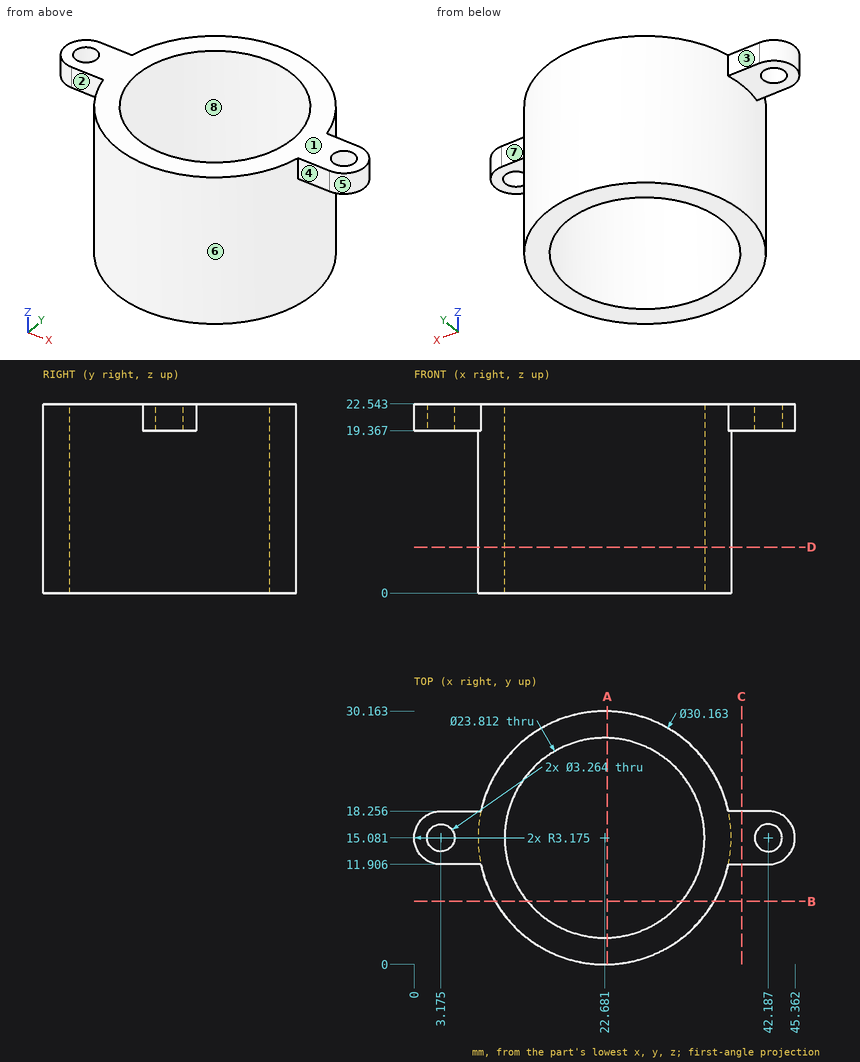
Answer from the drawing. Dimensions are ordinates in mm from the lowest x, y and z of the part. A direction names the side the tool comes from. Give positions to 0.01 mm unless a question says otherwise; leave off trailing zeros. Order: outer loops, then holes, each group sorted by start corner. A loop starts at its lowest first (then second) coordinate and runs counter-clockwise, first axis right, second up. Notation, with made-up numbers: (30.5, 40.5) -> (41.5, 40.5) arc R13 cw to (41.5, 52.5) -> close; hole circle Ø5 at (69, 39). An arc over 180 degrees is marked (long way). One line per item, written item: value.
Item 1: Find section A-A, the plane x = 23. Give the vertices of the cut face in (y, z), plus the area to 3 significant figures.
Answer sheet:
outline: (0, 0) -> (3.18, 0) -> (3.18, 22.54) -> (0, 22.54) -> close; (26.98, 0) -> (30.16, 0) -> (30.16, 22.54) -> (26.98, 22.54) -> close
area: 143 mm²
Item 2: Straight lines are drawn through the part: probe 1 along Y at (x, z) = (30.5, 12) (1 decimal); probe 2 along X at (y, z) = (16, 16.5) (1 decimal); probe 3 along X at (y, z) = (18.5, 1) (1 decimal). For each, find the intervals that lie inside material, in ascending order.
Answer sheet:
probe 1: 2.2 to 6.1, 24.1 to 28
probe 2: 7.6 to 10.8, 34.6 to 37.7
probe 3: 8 to 11.3, 34.1 to 37.4
Item 3: Find section D-D, the plane z = 5.5. Give the vertices of the cut face in (x, y).
Answer sheet:
outline: circle Ø30.16 at (22.68, 15.08); hole circle Ø23.81 at (22.68, 15.08)
Item 4: Find section C-C, the plane x = 39. Give the vertices of the cut face in (y, z).
Answer sheet:
outline: (11.91, 19.37) -> (18.26, 19.37) -> (18.26, 22.54) -> (11.91, 22.54) -> close
Item 5: A tool of negligible diameter and unlimited length cuts with its end or side. For the marked faces 1, 2, 3 and 4, from which of +Z, -Z, +X, -X, +Y, -Y can it reach the whole face along a straight path? Write none if from no direction.
Answer sheet:
face 1: +Z, +X, -X, +Y, -Y
face 2: +Z, -Z, -X, -Y
face 3: +Z, -Z, -X, +Y
face 4: +Z, -Z, +X, -Y
Item 6: Determine the mould class of the marked faces 5, 6, 7 and 8 for opening direction X: released by +X, released by -X, zero draft, split by the parting line, or undercut.
Answer sheet:
face 5: released by +X
face 6: split by the parting line
face 7: zero draft
face 8: undercut
Item 7: Flat-ended cylindrical pins translate along their axes: P1, Ø2.5, axis at x = 40, z = 20.5, coming from the -Y side; P2, Ø1, axis at y = 12, z = 6, coming from the +X side; P3, Ø1, axis at y = 8.5, z = 19.5, coming from the +X side; P4, Ø2.5, axis at x = 42.19, y = 15.08, coming from the -Z side. Find the tip coordinate at first contact, or state that the pin passes through.
Answer sheet:
P1: y = 11.91
P2: x = 37.54
P3: x = 36.48
P4: through
Item 8: Find section B-B, the plane y = 7.5. Give the vertices of the cut face in (x, z).
Answer sheet:
outline: (9.64, 0) -> (13.5, 0) -> (13.5, 22.54) -> (9.64, 22.54) -> close; (31.86, 0) -> (35.72, 0) -> (35.72, 22.54) -> (31.86, 22.54) -> close
